Design review of the part built by this model. Coordinates are the model's own, in mm. Face numbers are marked on the shaded views. Coordinates: 2 decimals unless noted, no trailing zeros. Loops run counter-clockwise (first coordinate to the right, second up) from the corner with the lowest first, then second, coordinate; pieces in that order, holes last. Notation, with made-up numbers: (17, 42) - (38, 42) arc R33 ccw to (38, 76) - close; hole circle Ø1 at (-17.75, 11.5). An arc over 180 degrees is marked (long way). Answer in a Markdown table with one row per item. Add a question column.
(1) Clearance check with flat-ended pins moving along their axes: pin 1 (7 mm diameter, centred on x = 0, y = -0.5, fed in from +Z); pin 2 (1.6 mm diameter, centred on x = 0, y = -0.5, fed in from -Z); pin 3 (1.5 mm diameter, centred on y = -4, z = 9, fed in from +X); pin 4 (3 mm diameter, centred on x = 2, z = 5, fed in from -Y). State where each tip first meets the part, or that it passes through.
(2) To check wall thickness, follow L1, parallel to Y at x = 0, z = 3.5 (3 decimals); L2, parallel to X at y = 0, z = -11. State the ranges of each line that lie inside material, in increasing order. Write a range as [from, to].
(3) The part is to be moulded in two halves that separate along Y. For the marked faces 1 and 2, say which applies: released by +Y, released by -Y, zero draft, split by the parting line, or undercut.
(4) We need section D-D, the plane y = -2.5. Write out the cut boundary in (x, z), plus the area to 3 significant figures.
(5) We need section C-C, the plane z = 8.5. Write out the cut boundary in (x, y) (3 decimals).
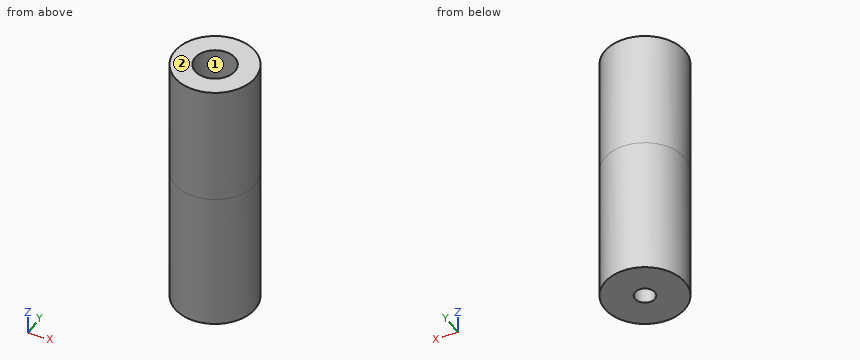
from build123d import *

# Parameters (mm, degrees)
F0_R     = 6.35
F0_R_2   = 3.175
F1_DEPTH = 14.2875
F2_R     = 6.35
F3_DEPTH = 4.7625
F4_R     = 6.35
F4_R_2   = 1.579033
F5_DEPTH = 22.225


with BuildPart() as f1:
    # F0 (on Top) → F1 (new body)
    with BuildSketch(Plane.XY):
        Circle(F0_R)
        Circle(F0_R_2, mode=Mode.SUBTRACT)
    extrude(amount=F1_DEPTH)

    # F2 (on face) → F3 (join)
    with BuildSketch(Plane.XY):
        Circle(F2_R)
    extrude(amount=-F3_DEPTH)

    # F4 (on face) → F5 (join)
    with BuildSketch(Plane(origin=(0, 0, -4.7625), x_dir=(1, 0, 0), z_dir=(0, 0, -1))):
        Circle(F4_R)
        Circle(F4_R_2, mode=Mode.SUBTRACT)
    extrude(amount=F5_DEPTH)


solid = f1.part
Responses:
| question | item | result |
|---|---|---|
| 1 | pin 1 | stops at z = 14.29 |
| 1 | pin 2 | stops at z = -4.76 |
| 1 | pin 3 | stops at x = 5.46 |
| 1 | pin 4 | stops at y = -6.33 |
| 2 | L1 | y = [-6.35, -3.175], [3.175, 6.35] |
| 2 | L2 | x = [-6.35, -1.58], [1.58, 6.35] |
| 3 | face 1 | undercut |
| 3 | face 2 | zero draft |
| 4 | outline | (-5.84, -26.99) - (5.84, -26.99) - (5.84, 14.29) - (1.96, 14.29) - (1.96, 0) - (-1.96, 0) - (-1.96, 14.29) - (-5.84, 14.29) - close |
| 4 | area | 426 mm2 |
| 5 | outline | circle Ø12.7 at (0, 0); hole circle Ø6.35 at (0, 0) |
